Autodesk Inventor part; units mm, degrees
ref_plane "YZ Plane" through (0, 0, 0) normal (1, 0, 0) x (0, 1, 0)
ref_plane "XZ Plane" through (0, 0, 0) normal (0, 1, 0) x (-1, 0, 0)
sketch "Sketch2" plane through (0, 0, 0) normal (0, 1, 0) x (-1, 0, 0)
  arc A0 (44.45, 506.057) -> (-44.45, 506.057) centre (0, -1.4242) ccw construction
  arc A1 (44.45, 506.057) -> (-44.45, 506.057) centre (0, -1.4242) ccw
  line L0 (44.45, 84.2423) -> (44.45, 506.057)
  line L1 (-44.45, 506.057) -> (-44.45, 84.2423)
  circle A2 centre (0, 0) radius 57.15 construction
  circle A3 centre (0, 0) radius 63.5
  arc A4 (-44.45, 84.2423) -> (44.45, 84.2423) centre (0, 0) ccw
  line L2 (0, 0) -> (0, 508) construction
  arc A5 (31.75, 494.2843) -> (-31.75, 494.2843) centre (0, -1.4242) ccw
  line L3 (-31.75, 494.2843) -> (-31.75, 69.85)
  arc A6 (-31.75, 77.0401) -> (31.75, 77.0401) centre (0, 0) ccw construction
  line L4 (31.75, 69.85) -> (31.75, 494.2843)
  arc A7 (31.75, 62.217) -> (-31.75, 62.217) centre (0, 0) ccw construction
  line L5 (0, 69.85) -> (0, 63.5) construction
  line L6 (-31.75, 69.85) -> (31.75, 69.85)
  point P0 (-7.0927, 251.5509)
  dimension "d23" = 127
  dimension "d21" = 88.9
  dimension "d22" = 114.3
  dimension "d24" = 190.5
  dimension "d25" = 508
  dimension "d26" = 88.9
  dimension "d29" = 12.7
  dimension "d31" = 139.7
  dimension "d69" = 12.7
  dimension "d70" = 12.7
extrude "Extrusion2" add sketch "Sketch2" along normal blind 12.7
sketch "Sketch3" plane through (0, 12.7, 0) normal (0, 1, 0) x (1, 0, 0)
  arc A0 (-44.4483, -506.0602) -> (44.4517, -506.0602) centre (0.0017, 1.4211) ccw construction
  line L0 (44.4517, -506.0602) -> (44.4517, -84.2454) construction
  line L1 (-44.4483, -506.0602) -> (44.4517, -506.0602) construction
  line L2 (44.4517, -506.0602) -> (44.4517, -84.2454) construction
  line L3 (44.4517, -84.2454) -> (-44.4483, -84.2454) construction
  line L4 (-44.4483, -84.2454) -> (-44.4483, -506.0602) construction
  line L5 (-44.4483, -84.2454) -> (-44.4483, -506.0602) construction
  line L6 (-44.4483, -295.1528) -> (-38.0983, -295.1528) construction
  line L7 (-38.0983, -295.1528) -> (-38.0983, -506.0602) construction
  line L8 (-38.0983, -295.1528) -> (-38.0983, -84.2454) construction
  circle A1 centre (-38.0983, -96.9454) radius 3.175
  circle A2 centre (-38.0983, -480.6602) radius 3.175
  circle A3 centre (-38.0983, -295.1528) radius 3.175
  line L9 (0.0017, -506.0602) -> (0.0017, 1.4211) construction
  circle A4 centre (38.1017, -295.1528) radius 3.175
  line L10 (44.4517, -295.1528) -> (38.1017, -295.1528) construction
  circle A5 centre (38.1017, -96.9454) radius 3.175
  circle A6 centre (38.1017, -480.6602) radius 3.175
  line L11 (38.1017, -295.1528) -> (38.1017, -506.0602) construction
  line L12 (38.1017, -295.1528) -> (38.1017, -84.2454) construction
  line L13 (44.4517, -84.2454) -> (44.4517, -506.0602) construction
  line L14 (44.4517, -84.2454) -> (44.4517, -506.0602) construction
  point P0 (0, 0)
  dimension "d54" = 6.35
  dimension "d55" = 90
  dimension "d56" = 6.35
  dimension "d57" = 12.7
  dimension "d58" = 6.35
  dimension "d59" = 6.35
  dimension "d60" = 25.4
extrude "Extrusion3" cut sketch "Sketch3" against normal blind 12.7
ref_plane "Work Plane2" through (0, 0, 494.411) normal (0, 0, 1) x (1, 0, 0)
sketch "Sketch5" plane through (0, 0, 494.411) normal (0, 0, 1) x (1, 0, 0)
  line L0 (-28.194, 25.4) -> (-28.194, 12.7) construction
  line L1 (-28.194, 25.4) -> (-15.494, 25.4) construction
  line L2 (-28.194, 12.7) -> (28.194, 12.7) construction
  line L3 (0, 12.7) -> (-28.194, 12.7) construction
  circle A0 centre (-14.097, 12.7) radius 6.35
  line L4 (0, 12.7) -> (0, 25.4) construction
  circle A1 centre (14.097, 12.7) radius 6.35
  line L5 (95.25, 12.7) -> (-95.25, 12.7) construction
  line L6 (95.25, 12.7) -> (-95.25, 12.7) construction
  line L7 (0, 12.7) -> (0, 0) construction
  line L8 (95.25, 0) -> (-95.25, 0) construction
  point P0 (44.45, 12.7)
  point P1 (44.45, 0)
  point P2 (-44.45, 0)
  dimension "d62" = 12.7
  dimension "d63" = 90
  dimension "d64" = 56.388
  dimension "d65" = 90
  dimension "d66" = 12.7
extrude "Extrusion5" cut sketch "Sketch5" along normal blind 6.35
equation "\"d26\" = d21"
properties part number "Arm Layer 2"
Design review of the part built by this model. Coordinates are the model's own, in mm. A direction names the side the tool comes from. Give positions to 0.01 mm unless a question says otherwise; leave off trailing zeros. Write each loop counter-clockwise with the first axis right and the second up, starting at its lowest first coordinate (ties: lowest second). Pieces come first, ordered by that corner, then holes. Notation, with made-up numbers: (39, 42.5) - (94, 42.5) arc R16 cw to (94, 63.5) - close; hole circle Ø9 at (6.5, 85.5). An arc over 180 degrees is marked (long way). Return JSON: item names as keys, results as strings. Group by question number.
(1) To check wall thickness, follow probe 1 along X at (y, z) = (6.75, 280); probe 2 along Z at (x, y) = (8, 2.25); probe 3 along X at (y, z) = (9.5, 298). State the ranges of each line that lie inside material, in increasing order.
(2) Insertion check: pin 1 (6.5 mm diameter, centred on y = 4, z = 345.5, fed in from +X); pin 2 (1 mm diameter, centred on y = 1.5, z = 264.5, fed in from -X); pin 3 (5 mm diameter, centred on x = 16.5, y = 9.5, fed in from -Z); pin 4 (5.5 mm diameter, centred on x = 38.1, z = 96.95, fed in from -Y). Each pin has a flat end and moves straight along its axis. Give the tip position at first contact, or say it passes through.
(3) We need section D-D, the plane z = 77. Give the boundary of the cut face in (x, y), then the cut area to 3 significant figures.
(4) We need section C-C, the plane y = 2.5. Give the number of separate pieces and of enclosed holes in the cut face, then the cut area to 3 significant figures.
(5) Mouldability with a two-part tool opening along Z and no side actions: class faces 4 (the flat face through (31.75, 6, 285)), 5 (the cylindrical face through (-3.541, 6.261, -95.184)), 6 (the cylindrical face through (1, 6, 508)), 7 (the flat face through (44.45, 6, 298)) as +Z half, -Z half, draft (parallel to the pull), parting line (faces both ways), or undercut.
(6) Machinability: for faces 1 (the flat face through (36, 12.7, 141)), 2 (the flat face through (-31.75, 6, 279)), 3 (the flat face through (-44.45, 6, 292)), which of the approach directions +Z, -Z, +X, -X, +Y, -Y give a long, thin tool a straight path to every point of the face, cutting with its end or side? Answer none if there is none.
(7) We need section A-A, the plane x = 0. Give the boundary of the cut face in (y, z).
(8) We need section B-B, the plane z = 191.5. Give the boundary of the cut face in (x, y).
Reported:
{
 "1": {"probe 1": "x = -44.45 to -31.75, 31.75 to 44.45", "probe 2": "z = -94.91 to -62.99, 62.99 to 69.85, 495.24 to 507.94", "probe 3": "x = -44.45 to -39.5, -36.69 to -31.75, 31.75 to 36.7, 39.51 to 44.45"},
 "2": {"pin 1": "stops at x = 44.45", "pin 2": "stops at x = -44.45", "pin 3": "stops at z = -94.22", "pin 4": "passes through"},
 "3": {"outline": "(-56.07, 0) - (-31.75, 0) - (-31.75, 12.7) - (-56.07, 12.7) - close; (31.75, 0) - (56.07, 0) - (56.07, 12.7) - (31.75, 12.7) - close", "area": "618 mm2"},
 "4": {"separate pieces": "1", "enclosed holes": "8", "area": "25,600 mm2"},
 "5": {"face 4": "undercut", "face 5": "parting line", "face 6": "+Z half", "face 7": "draft"},
 "6": {"face 1": "+Z, -Z, +X, -X, +Y", "face 2": "+Y, -Y", "face 3": "+Z, -X, +Y, -Y"},
 "7": {"outline": "(0, -95.25) - (12.7, -95.25) - (12.7, -63.5) - (0, -63.5) - close; (0, 63.5) - (12.7, 63.5) - (12.7, 69.85) - (0, 69.85) - close; (0, 495.3) - (12.7, 495.3) - (12.7, 508) - (0, 508) - close"},
 "8": {"outline": "(-44.45, 0) - (-31.75, 0) - (-31.75, 12.7) - (-44.45, 12.7) - close; (31.75, 0) - (44.45, 0) - (44.45, 12.7) - (31.75, 12.7) - close"}
}
